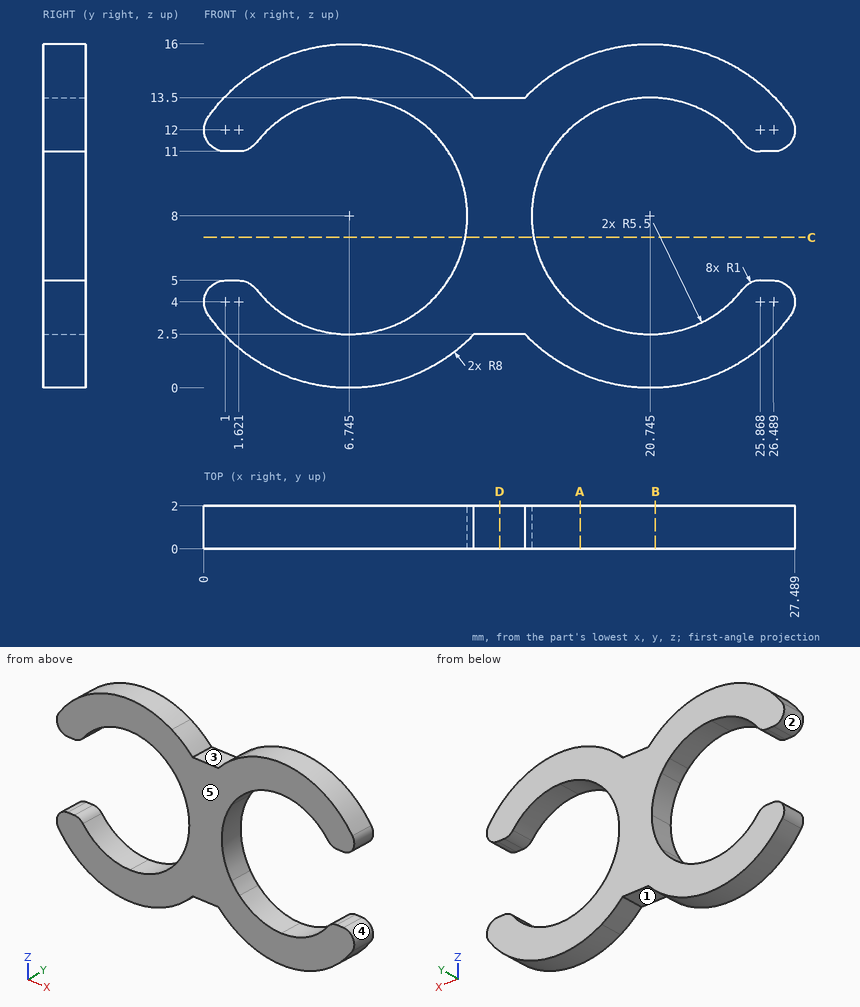
Can you work these out from the drawing? Everything is in mm from the part's minimum corner. A direction names the side the tool comes from. Round coordinates to 2 decimals unless told otherwise and drop trailing zeros. Loops run counter-clockwise (first coordinate to the right, second up) from the corner with the lowest first, then second, coordinate; pieces in that order, holes last. Notation, with made-up numbers: (24, 33) - (78, 33) arc R22 cw to (78, 72) - close; hole circle Ø7 at (-37.5, -32.75). An arc over 180 degrees is marked (long way). Write item = value, one per line. Start each with the question number.
(1) If we section it at A-A (x = 17.5): Please give me the cut outline in (y, z).
(2) If we section it at D-D (x = 13.75): Please give me the cut outline in (y, z), and give its area (3 significant figures).
(3) If we section it at C-C (z = 7): Please give me the cut outline in (x, y).
(4) If I drill on probe 1 along X at (y, z) = (0.9, 12); probe 2 along X at (y, z) = (0.35, 12.5) (1 decimal); probe 3 along X at (y, z) = (1.05, 2) (1 decimal), over which ranges is the centre line in solid material (lowest first)? Write a range as [from, to].
(5) If we mould it in two halves opening along X, with no side actions, what happens to the marked faces 3, 4 and 5? For each: released by +X, released by -X, zero draft, split by the parting line, or undercut.
(6) For the marked faces 1 and 2, which set-ups out of +Z, -Z, +X, -X, +Y, -Y let a thin tool reach every point of the face, with its end or its side?
(7) For P1, Ø0.5, axis at x = 26, y = 1, coming from the -Z side; P2, Ø0.7, axis at x = 1, y = 1, coming from the +Z side; P3, Ø0.6, axis at x = 13.5, y = 1, coming from the -Z side; P4, Ø3, axis at x = 4, z = 13.5, coming from the -Y side, each with a flat end and sliding along its axis, tell me the tip position at first contact or that it passes through.
(8) If we section it at B-B (x = 21): Please give me the cut outline in (y, z).
Ans:
q1.outline = (0, 0.69) - (2, 0.69) - (2, 3.56) - (0, 3.56) - close; (0, 12.44) - (2, 12.44) - (2, 15.31) - (0, 15.31) - close
q2.outline = (0, 2.5) - (2, 2.5) - (2, 13.5) - (0, 13.5) - close
q2.area = 22.0 mm²
q3.outline = (12.15, 0) - (15.34, 0) - (15.34, 2) - (12.15, 2) - close
q4.probe_1 = [0, 2.97], [10.52, 16.97], [24.52, 27.49]
q4.probe_2 = [0.1, 3.6], [9.9, 17.6], [23.9, 27.4]
q4.probe_3 = [1.5, 12], [15.5, 26]
q5.face_3 = undercut
q5.face_4 = released by +X
q5.face_5 = zero draft
q6.face_1 = -Z, +Y, -Y
q6.face_2 = -X, +Y, -Y
q7.P1 = 1.76
q7.P2 = 13.91
q7.P3 = 2.5
q7.P4 = 0
q8.outline = (0, 0) - (2, 0) - (2, 2.51) - (0, 2.51) - close; (0, 13.49) - (2, 13.49) - (2, 16) - (0, 16) - close
